The listing builds one solid part. Answer for the finished solid, in the listing's coordinates (mm). Give positions to 0.01 mm unless a question says otherwise; leave off trailing zeros. Loops run counter-clockwise (first coordinate to the right, second up) from the corner with the lowest first, then second, coordinate; pieces in that order, holes last. Notation, with made-up numbers: M 27.25,-38 L 40.25,-38 A19 ccw 40.25,-22 Z; hole C 73.25,31 d1. An arc over 180 degrees is marked long. One line per item, written item: value. Start each with the question number.
Q1. A cutting plane is placed at A-A, the plane x = 0. Determine the outline of the cut face in (y, z), and give its area (3 significant figures).
Q2. Consider L1, parallel to X at y = 0.35, z = -5; L2, parallel to Z at x = 3.5, y = 1.4; L3, parallel to X at y = 1.55, z = 19.5. Determine where each line is inside the solid, lowest interval first.
Q3. Flat-ended cylindrical pins translate along their axes: pin 1 (6 mm diameter, centred on x = -5.02, z = 32.11, fed in from +Y); pin 2 (1 mm diameter, centred on y = 1, z = -5.5, fed in from +X); pin 3 (1 mm diameter, centred on x = 6, y = 0.5, fed in from -Z); pin 4 (4 mm diameter, centred on x = 5.02, z = -32.11, fed in from -Y). Find the tip coordinate at first contact, or state that the pin passes through.
Q4. A cutting plane is placed at C-C, the plane y = 0.5. State how many separate pieces and enclosed holes the cut face has, and give its area (3 significant figures).
Q5. A cutting plane is placed at B-B, the plane z = 0. Determine the outline of the cut face in (x, y).
Q6. The mould has two halves that part along X. Classify faces 1 (the cylindrical face through (-24.397, 0.986, 12.69)), 2 (the cylindrical face through (-5.61, 0.99, 29.68)), 3 (the cylindrical face through (-39.05, 0.99, -8.67)), 4 (the flat face through (-26.1, 0, -9.4)): +X half, -X half, draft (parallel to the pull), parting line (faces both ways), or undercut.
from build123d import *

# Parameters (mm, degrees)
SKETCH_1_R          = 40
SKETCH_1_R_2        = 27.5
EXTRUDE_1_DEPTH     = 2
CUT_EXTRUDE_1_DEPTH = 5


with BuildPart() as part:
    # 草图1 → 凸台-拉伸1 (new body)
    with BuildSketch(Plane(origin=(0, 0, 0), x_dir=(1, 0, 0), z_dir=(0, 1, 0))):
        with Locations(Location((0, 0, 0), (0, 0, 270))):
            Circle(SKETCH_1_R)
        with Locations(Location((0, 0, 0), (0, 0, 270))):
            Circle(SKETCH_1_R_2, mode=Mode.SUBTRACT)
    extrude(amount=EXTRUDE_1_DEPTH)

    # 草图2 → 切除-拉伸1 (cut)
    with BuildSketch(Plane.XZ):
        with BuildLine():
            ThreePointArc((-32.496342046, -2.547106912), (-34.580439739, -5.403072039), (-31.724474612, -7.487169732))
            ThreePointArc((-31.724474612, -7.487169732), (-29.640376919, -4.631204605), (-32.496342046, -2.547106912))
        make_face()
        with BuildLine():
            ThreePointArc((-26.639073723, 21.627866356), (-28.723171416, 18.771901229), (-25.867206289, 16.687803537))
            ThreePointArc((-25.867206289, 16.687803537), (-23.783108596, 19.543768664), (-26.639073723, 21.627866356))
        make_face()
        with BuildLine():
            ThreePointArc((-5.403072039, 34.580439739), (-7.487169732, 31.724474612), (-4.631204605, 29.640376919))
            ThreePointArc((-4.631204605, 29.640376919), (-2.547106912, 32.496342046), (-5.403072039, 34.580439739))
        make_face()
        with BuildLine():
            ThreePointArc((18.771901229, 28.723171416), (16.687803537, 25.867206289), (19.543768664, 23.783108596))
            ThreePointArc((19.543768664, 23.783108596), (21.627866356, 26.639073723), (18.771901229, 28.723171416))
        make_face()
        with BuildLine():
            ThreePointArc((31.724474612, 7.487169732), (29.640376919, 4.631204605), (32.496342046, 2.547106912))
            ThreePointArc((32.496342046, 2.547106912), (34.580439739, 5.403072039), (31.724474612, 7.487169732))
        make_face()
        with BuildLine():
            ThreePointArc((25.867206289, -16.687803537), (23.783108596, -19.543768664), (26.639073723, -21.627866356))
            ThreePointArc((26.639073723, -21.627866356), (28.723171416, -18.771901229), (25.867206289, -16.687803537))
        make_face()
        with BuildLine():
            ThreePointArc((-19.543768664, -23.783108596), (-21.627866356, -26.639073723), (-18.771901229, -28.723171416))
            ThreePointArc((-18.771901229, -28.723171416), (-16.687803537, -25.867206289), (-19.543768664, -23.783108596))
        make_face()
        with BuildLine():
            ThreePointArc((4.631204605, -29.640376919), (2.547106912, -32.496342046), (5.403072039, -34.580439739))
            ThreePointArc((5.403072039, -34.580439739), (7.487169732, -31.724474612), (4.631204605, -29.640376919))
        make_face()
    extrude(amount=-CUT_EXTRUDE_1_DEPTH, mode=Mode.SUBTRACT)


solid = part.part
Answer block:
1. outline: M 0,-40 L 2,-40 L 2,-27.5 L 0,-27.5 Z; M 0,27.5 L 2,27.5 L 2,40 L 0,40 Z
1. area: 50.0 mm^2
2. L1: -39.69 to -34.61, -29.61 to -27.04, 27.04 to 39.69
2. L2: -39.85 to -34.1, -30.12 to -27.28, 27.28 to 39.85
2. L3: -34.92 to -28.73, -23.78 to -19.39, 19.39 to 34.92
3. pin 1: y = 2
3. pin 2: x = 39.69
3. pin 3: z = -39.62
3. pin 4: through
4. separate pieces: 1
4. enclosed holes: 9
4. area: 2,490 mm^2
5. outline: M -40,0 L -27.5,0 L -27.5,2 L -40,2 Z; M 27.5,0 L 40,0 L 40,2 L 27.5,2 Z
6. face 1: undercut
6. face 2: undercut
6. face 3: parting line
6. face 4: draft
